Verification items for the finished model (mm, model axes). A direction names the side the tool comes from. Round coordinates to 2 decimals unless told otherwise and drop trailing zeros. Order: outer loops, then holes, each group sorted by start corner. A loop starts at its lowest first (then second) coordinate and runs counter-clockwise, first axis right, second up. Notation, with made-up numbers: (56.25, -35) -> (88.25, -35) arc R19 cw to (88.25, -17) -> close; hole circle Ø11 at (-24.75, 70). An arc over 180 degrees is marked (long way). Return JSON: item names as keys, results as strings. Group by question number.
Item 1: Depth check by flat-ended pin: pin 1 Ø2 at (x, z) = (0.5, -3) entering from +Y; pin 2 Ø1.7 at (x, y) = (1, 1) entering from +Z; pin 3 Ø1.5 at (y, z) = (6.5, -2.5) entering from +X; pin 4 Ø3 at (x, z) = (-3, -7) entering from +Y. Enter the tip coordinate at first touch or a pass-through.
Item 2: Draft check along Z on faces 1 (the flat face through (4, 0, -6)), 2 (the flat face through (5.849, 0.805, -12.185)), 3 (the flat face through (1, 1, -8.661)). Enter one of: pulls with the +Z half, pulls with the -Z half, needs draft (parallel to the pull), parting line crosses it, or undercut.
Item 3: Sectioned sample at A-A on x = 0. Record the cut outline in (y, z), plus the area to 3 significant figures.
Item 4: Sectioned sample at C-C on z = -1.5. Record the cut outline in (x, y), plus the area to 3 significant figures.
Item 5: Access from +Z, -Z, +X, -X, +Y, -Y to the whole of each face (thin tool, end or side, straight path). Record for faces 4 (the flat face through (1, 1, -4.039)), 5 (the flat face through (-4.762, 5, -6)), 6 (the flat face through (-6, 9.83, -6)).
Item 6: Sectioned sample at D-D on x = -5. Record the cut outline in (y, z) (3 decimals).
Item 7: Sectioned sample at B-B on y = 8.75. Record the cut outline in (x, z).
Item 8: Scan lines: probe 1 along Y at (x, z) = (3.25, -10.5); probe 2 along X at (y, z) = (9.75, -2.25); probe 3 along X at (y, z) = (2, -9.25). Record each from-to range of solid material in increasing order. Write a range as from..to.
Autodesk Inventor part; units mm, degrees
ref_plane "Diagonal Plane" through (-4.7625, 1.5875, 0) normal (-0.7071068, 0.7071068, 0) x (0, 0, 1)
ref_plane "YZ Plane" through (0, 0, 0) normal (1, 0, 0) x (0, 1, 0)
ref_plane "XZ Plane" through (0, 0, 0) normal (0, 1, 0) x (-1, 0, 0)
sketch "Sketch1" plane through (0, 0, 0) normal (0, 1, 0) x (-1, 0, 0)
  line L0 (-6.35, 0) -> (6.35, 0)
  line L1 (6.35, 0) -> (6.35, -12.7)
  line L2 (6.35, -12.7) -> (-6.35, -12.7)
  line L3 (-6.35, -12.7) -> (-6.35, 0)
  line L4 (6.35, 0) -> (-6.35, -12.7) construction
  point P0 (0, 0)
  point P1 (0, 0)
  dimension "d0" = 12.7
  dimension "d1" = 12.7
extrude "Plate1" add sketch "Sketch1" along normal blind 1.5875
sketch "Sketch2" plane through (-4.7625, 0, 0) normal (-1, 0, 0) x (0, -1, 0)
  line L0 (0, -12.7) -> (0, 0)
  line L1 (0, 0) -> (-12.7, 0)
  line L2 (-12.7, 0) -> (-12.7, -12.7)
  line L3 (-12.7, -12.7) -> (0, -12.7)
edge flange "Flanges" height 12.7 angle 90 thickness 1.5875 bend radius 0.7937 thickness toward (-1, 0, 0) relief tear relief width 1.5875 relief depth 0.7937 edges at (-6.35, 1.5875, -6.35) wall of the first edge with corners at (-4.7625, 0, -12.7) (-4.7625, 0, 0) (-4.7625, 12.7, 0) (-4.7625, 12.7, -12.7)
bend "Bend1"
corner "Corner1"
sketch "Sketch8" plane through (0, 0, 0) normal (0, -1, 0) x (1, 0, 0)
  line L0 (6.35, 0) -> (-3.9687, 0) construction
  line L1 (2.9718, -4.0386) -> (-0.635, -4.0386)
  line L2 (-1.143, -4.5466) -> (-1.143, -8.1534)
  line L3 (-0.635, -8.6614) -> (2.9718, -8.6614)
  line L4 (3.4798, -8.1534) -> (3.4798, -4.5466)
  arc A0 (3.4798, -4.5466) -> (2.9718, -4.0386) centre (2.9718, -4.5466) ccw
  arc A1 (2.9718, -8.6614) -> (3.4798, -8.1534) centre (2.9718, -8.1534) ccw
  arc A2 (-1.143, -8.1534) -> (-0.635, -8.6614) centre (-0.635, -8.1534) ccw
  arc A3 (-0.635, -4.0386) -> (-1.143, -4.5466) centre (-0.635, -4.5466) ccw
  line L5 (2.9718, -4.5466) -> (-0.635, -8.1534) construction
  line L6 (6.35, -12.7) -> (6.35, 0) construction
  point P0 (0, 0)
  point P1 (-1.143, -8.6614)
  point P2 (3.4798, -8.6614)
  point P3 (12.7, 0)
  point P4 (1.1684, -6.35)
  dimension "d49" = 4.6228
  dimension "d50" = 0.508
  dimension "d52" = 6.35
  dimension "d123" = 5.1816
extrude "Body Stamp" cut sketch "Sketch8" against normal blind 1.5875
sketch "Sketch9" plane through (0, 0, 0) normal (0, -1, 0) x (1, 0, 0)
  arc A0 (3.4798, -4.5466) -> (2.9718, -4.0386) centre (2.9718, -4.5466) ccw construction
  arc A1 (-1.143, -8.1534) -> (-0.635, -8.6614) centre (-0.635, -8.1534) ccw construction
  line L0 (2.9718, -4.5466) -> (-0.635, -8.1534) construction
  circle A2 centre (1.1684, -6.35) radius 2.1844
  point P0 (0, 0)
  dimension "d55" = 4.3688
surface extrude "Body Circle" sketch "Sketch9" against normal up to surface (1.5875 mm away) shown yes curves A2
pattern_sketch "Body Pattern" of "Body Stamp", "Body Circle" from (1.1684, 0, -6.35) copies at (1.1684, 0, -19.05) at (1.1684, 0, -31.75) at (1.1684, 0, -44.45) at (1.1684, 0, -57.15) at (1.1684, 0, -69.85) at (1.1684, 0, -82.55) at (1.1684, 0, -95.25) at (1.1684, 0, -107.95) at (1.1684, 0, -120.65) at (1.1684, 0, -133.35) at (1.1684, 0, -146.05) at (1.1684, 0, -158.75) at (1.1684, 0, -171.45) at (1.1684, 0, -184.15) at (1.1684, 0, -196.85) at (1.1684, 0, -209.55) at (1.1684, 0, -222.25) at (1.1684, 0, -234.95) at (1.1684, 0, -247.65) at (1.1684, 0, -260.35) at (1.1684, 0, -273.05) at (1.1684, 0, -285.75) at (1.1684, 0, -298.45) at (1.1684, 0, -311.15) at (1.1684, 0, -323.85) at (1.1684, 0, -336.55) at (1.1684, 0, -349.25) at (1.1684, 0, -361.95) at (1.1684, 0, -374.65) at (1.1684, 0, -387.35) at (1.1684, 0, -400.05) at (1.1684, 0, -412.75) at (1.1684, 0, -425.45) at (1.1684, 0, -438.15)
sketch "Arc Length" plane through (19.05, 2.3812, 0) normal (0, 0, 1) x (1, 0, 0)
  line L0 (-25.4, 0) -> (-23.8125, 0)
  arc A0 (-25.4, 0) -> (-23.0187, -2.3813) centre (-23.0187, 0) ccw
  line L1 (-23.0187, -0.7938) -> (-23.0187, -2.3813)
  arc A1 (-23.8125, 0) -> (-23.0187, -0.7938) centre (-23.0187, 0) ccw
  point P0 (-19.05, -2.3812)
  dimension "d126" = 1.2468
  dimension "d127" = 3.7405
feature "Notch" [suppressed]
pattern_linear "Notch Pattern" [suppressed]
ref_plane "Diagonal Plane" through (-4.7625, 1.5875, 0) normal (-0.7071068, 0.7071068, 0) x (0, 0, 1)
mirror "Everything Mirrored" about plane through (-4.7625, 1.5875, 0) normal (-0.7071068, 0.7071068, 0) of "Body Stamp", "Body Circle", "Body Pattern"
chamfer "End Chamfer" distance 1.016 angle 45 4 edges at (-5.5562, 12.7, -12.7) (-5.5562, 12.7, 0) (6.35, 0.7937, 0) (6.35, 0.7937, -12.7)
sketch "Body Pattern Sketch" plane through (0, 0, 0) normal (0, -1, 0) x (1, 0, 0)
  line L0 (1.1684, -6.35) -> (1.1684, 0) construction
  circle A0 centre (1.1684, -6.35) radius 2.1844 construction
  point P0 (1.1684, -19.05)
  point P1 (1.1684, -31.75)
  point P2 (1.1684, -44.45)
  point P3 (1.1684, -57.15)
  point P4 (1.1684, -69.85)
  point P5 (1.1684, -82.55)
  point P6 (1.1684, -95.25)
  point P7 (1.1684, -107.95)
  point P8 (1.1684, -120.65)
  point P9 (1.1684, -133.35)
  point P10 (1.1684, -146.05)
  point P11 (1.1684, -158.75)
  point P12 (1.1684, -171.45)
  point P13 (1.1684, -184.15)
  point P14 (1.1684, -196.85)
  point P15 (1.1684, -209.55)
  point P16 (1.1684, -222.25)
  point P17 (1.1684, -234.95)
  point P18 (1.1684, -247.65)
  point P19 (1.1684, -260.35)
  point P20 (1.1684, -273.05)
  point P21 (1.1684, -285.75)
  point P22 (1.1684, -298.45)
  point P23 (1.1684, -311.15)
  point P24 (1.1684, -323.85)
  point P25 (1.1684, -336.55)
  point P26 (1.1684, -349.25)
  point P27 (1.1684, -361.95)
  point P28 (1.1684, -374.65)
  point P29 (1.1684, -387.35)
  point P30 (1.1684, -400.05)
  point P31 (1.1684, -412.75)
  point P32 (1.1684, -425.45)
  point P33 (1.1684, -438.15)
  dimension "d133" = 12.7
sketch "Sketch13" plane through (-6.35, 0, 431.8) normal (1, 0, 0) x (0, 0, -1)
  line L0 (493.268, 12.7) -> (495.3, 10.668)
  line L1 (495.3, 10.668) -> (497.332, 12.7)
  line L2 (493.268, 12.7) -> (497.332, 12.7)
  line L3 (495.3, 3.3973) -> (493.0372, 1.1344)
  line L4 (493.0372, 1.1344) -> (495.3, -1.1284)
  line L5 (495.3, -1.1284) -> (497.5628, 1.1344)
  line L6 (497.5628, 1.1344) -> (495.3, 3.3973)
  line L7 (495.3, 3.3973) -> (495.3, -1.1284) construction
  line L8 (495.3, 10.668) -> (495.3, 3.3973) construction
  line L9 (444.5, 12.7) -> (431.8, 12.7)
  line L10 (444.5, 2.3813) -> (431.8, 2.3813) construction
  line L11 (431.8, 12.7) -> (431.8, 2.3813) construction
  point P0 (444.5, -11.9062)
  point P1 (431.8, 0)
  dimension "d86" = 4.5256
  dimension "d128" = 2.032
  dimension "d129" = 1.016
  dimension "d130" = 63.5
equation "\"d53\" = Thickness"
equation "\"d89\" = Thickness"
equation "\"d1\" = 1.27 * Length"
equation "\"d2\" = Thickness"
equation "\"d3\" = BendReliefWidth"
equation "\"d4\" = BendReliefDepth"
equation "\"d5\" = MinimumRemnant"
equation "\"d6\" = TransitionRadius"
equation "\"d10\" = CornerReliefSize"
equation "\"d11\" = GapSize"
equation "\"d12\" = JacobiRadiusSize"
equation "\"BendRadius\" = Thickness"
equation "\"BendReliefWidth\" = Thickness"
equation "\"BendReliefDepth\" = 0.5 * Thickness"
equation "\"CornerReliefSize\" = 4 * Thickness"
equation "\"MinimumRemnant\" = 2 * Thickness"
equation "\"TransitionRadius\" = BendRadius"
equation "\"JacobiRadiusSize\" = BendRadius"
equation "\"GapSize\" = Thickness"
properties part number "Alu C 1x2x1x35"
Recorded:
{
 "1": {"pin 1": "y = 1.59", "pin 2": "z = 0", "pin 3": "x = -4.76", "pin 4": "y = 1.79"},
 "2": {"face 1": "needs draft", "face 2": "pulls with the -Z half", "face 3": "undercut"},
 "3": {"outline": "(0, -12.7) -> (1.59, -12.7) -> (1.59, -8.66) -> (0, -8.66) -> close; (0, -4.04) -> (1.59, -4.04) -> (1.59, 0) -> (0, 0) -> close", "area": "12.8 mm²"},
 "4": {"outline": "(-6.35, 2.38) arc R2.38 ccw to (-3.97, 0) -> (6.35, 0) -> (6.35, 1.59) -> (-3.97, 1.59) arc R0.79 cw to (-4.76, 2.38) -> (-4.76, 12.7) -> (-6.35, 12.7) -> close", "area": "36.7 mm²"},
 "5": {"face 4": "+Y, -Y", "face 5": "+Z, -Z, +X, +Y", "face 6": "+X, -X"},
 "6": {"outline": "(0.235, -12.7) -> (11.684, -12.7) -> (12.7, -11.684) -> (12.7, -1.016) -> (11.684, 0) -> (0.235, 0) -> close; hole (5.207, -8.153) arc R0.508 ccw to (5.715, -8.661) -> (9.322, -8.661) arc R0.508 ccw to (9.83, -8.153) -> (9.83, -4.547) arc R0.508 ccw to (9.322, -4.039) -> (5.715, -4.039) arc R0.508 ccw to (5.207, -4.547) -> close"},
 "7": {"outline": "(-6.35, -12.7) -> (-4.76, -12.7) -> (-4.76, -8.66) -> (-6.35, -8.66) -> close; (-6.35, -4.04) -> (-4.76, -4.04) -> (-4.76, 0) -> (-6.35, 0) -> close"},
 "8": {"probe 1": "0..1.59", "probe 2": "-6.35..-4.76", "probe 3": "-6.32..-4.66"}
}
